Here's the drawing with two shaded views (mm, measured from the low corner). I have some questions. Coordinates: 2 decimals unless noted, no trailing zeros. Loops run counter-clockwise (first coordinate to the right, second up) from the corner with the lowest first, then second, coordinate; pieces in that order, holes last. Notation, with made-up numbers: (-31.75, 53) -> (-22.75, 53) arc R8 cw to (-22.75, 65) -> close; hole circle Ø8 at (-26, 7.25). An arc over 180 degrees is marked (long way). Answer as a JSON object with one key per item and string values. Group by question number.
1) If we mould it in two halves opening along X, with no side actions, what happens to the marked faces 1, 2, 3 and 4? For each: +X half, -X half, draft (parallel to the pull), parting line (faces both ways), or undercut.
2) I'm going to push flat-ended pins straight in: pin 1 (3 mm diameter, centred on y = 11, z = 10.5, fed in from -X); pin 2 (5 mm diameter, centred on x = 10, z = 10, fed in from +Y). Where does each tip first touch, or does it pass through?
3) I need wall thicknesses on probe 1 along X at (y, z) = (9.5, 10); probe 2 along X at (y, z) = (11.25, 10) (1 decimal); probe 3 along X at (y, z) = (15.75, 9.5) (1 decimal). Which ranges of each line are inside material? Lowest first, please. Write a range as [from, to].
4) I want a section at A-A (y = 10). Write out the boundary of the cut face in (x, z), then the cut area to 3 significant figures.
5) I want a section at C-C (z = 10). Write out the boundary of the cut face in (x, y), then the cut area to 3 significant figures.
6) I want a section at D-D (y = 14.5). Write out the boundary of the cut face in (x, z).
7) I want a section at B-B (x = 70). Write out the boundary of the cut face in (y, z).
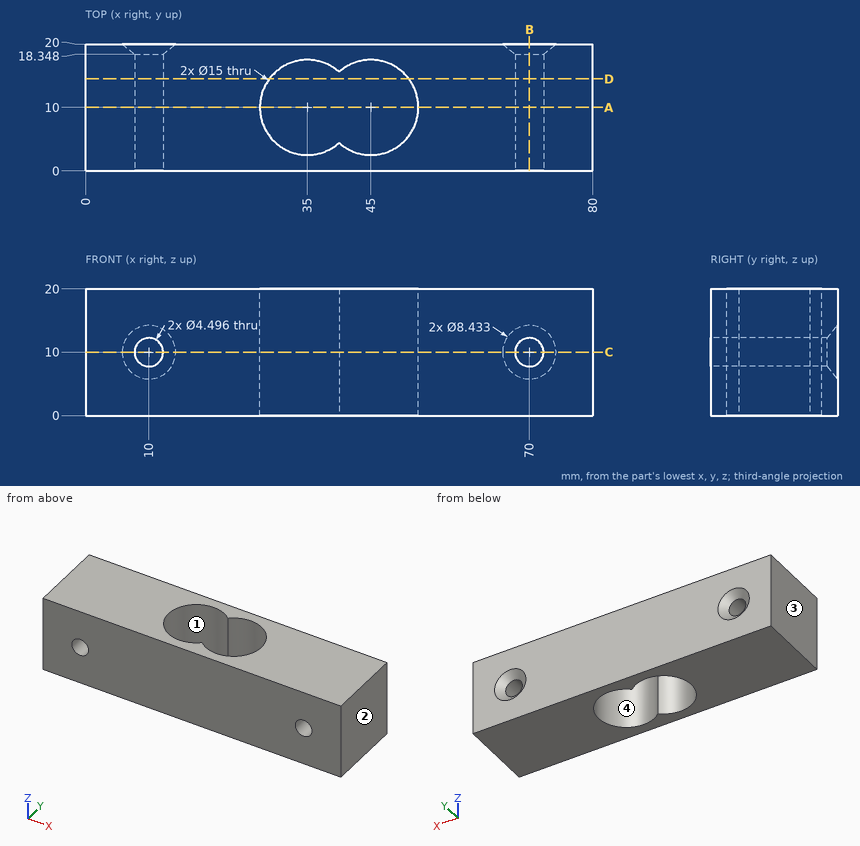
Determined:
{
 "1": {"face 1": "undercut", "face 2": "+X half", "face 3": "-X half", "face 4": "undercut"},
 "2": {"pin 1": "x = 0", "pin 2": "y = 18.56"},
 "3": {"probe 1": "[0, 7.75], [12.25, 27.52], [52.48, 67.75], [72.25, 80]", "probe 2": "[0, 7.8], [12.2, 27.6], [52.4, 67.8], [72.2, 80]", "probe 3": "[0, 7.8], [12.2, 30.2], [39.8, 40.2], [49.8, 67.8], [72.2, 80]"},
 "4": {"outline": "(0, 0) -> (27.5, 0) -> (27.5, 20) -> (0, 20) -> close; (52.5, 0) -> (80, 0) -> (80, 20) -> (52.5, 20) -> close; hole circle Ø4.5 at (10, 10); hole circle Ø4.5 at (70, 10)", "area": "1,070 mm^2"},
 "5": {"outline": "(0, 0) -> (7.75, 0) -> (7.75, 18.35) -> (5.78, 20) -> (0, 20) -> close; (12.25, 0) -> (67.75, 0) -> (67.75, 18.35) -> (65.78, 20) -> (14.22, 20) -> (12.25, 18.35) -> close; (72.25, 0) -> (80, 0) -> (80, 20) -> (74.22, 20) -> (72.25, 18.35) -> close; hole (40, 4.41) arc R7.5 ccw (long way) to (40, 15.59) arc R7.5 ccw (long way) to start", "area": "1,100 mm^2"},
 "6": {"outline": "(0, 0) -> (29, 0) -> (29, 20) -> (0, 20) -> close; (51, 0) -> (80, 0) -> (80, 20) -> (51, 20) -> close; hole circle Ø4.5 at (10, 10); hole circle Ø4.5 at (70, 10)"},
 "7": {"outline": "(0, 0) -> (20, 0) -> (20, 5.78) -> (18.35, 7.75) -> (0, 7.75) -> close; (0, 12.25) -> (18.35, 12.25) -> (20, 14.22) -> (20, 20) -> (0, 20) -> close"}
}
